For this review, use the dimensioned drawing (mm, ordinates from the lowest corner) and the shaded views. A direction names the side the tool comes from. Coordinates: 2 decimals unless noted, no trailing zeros. Loops run counter-clockwise (first coordinate to the right, second up) from the corner with the lowest first, then second, coordinate; pieces in that order, holes last. Notation, with made-up numbers: M -10.75,12.25 L 14.25,12.25 A28 cw 14.25,39.25 Z; hole C 88.25,72 d3. An arc over 180 degrees is marked long. One line per item, written item: value.
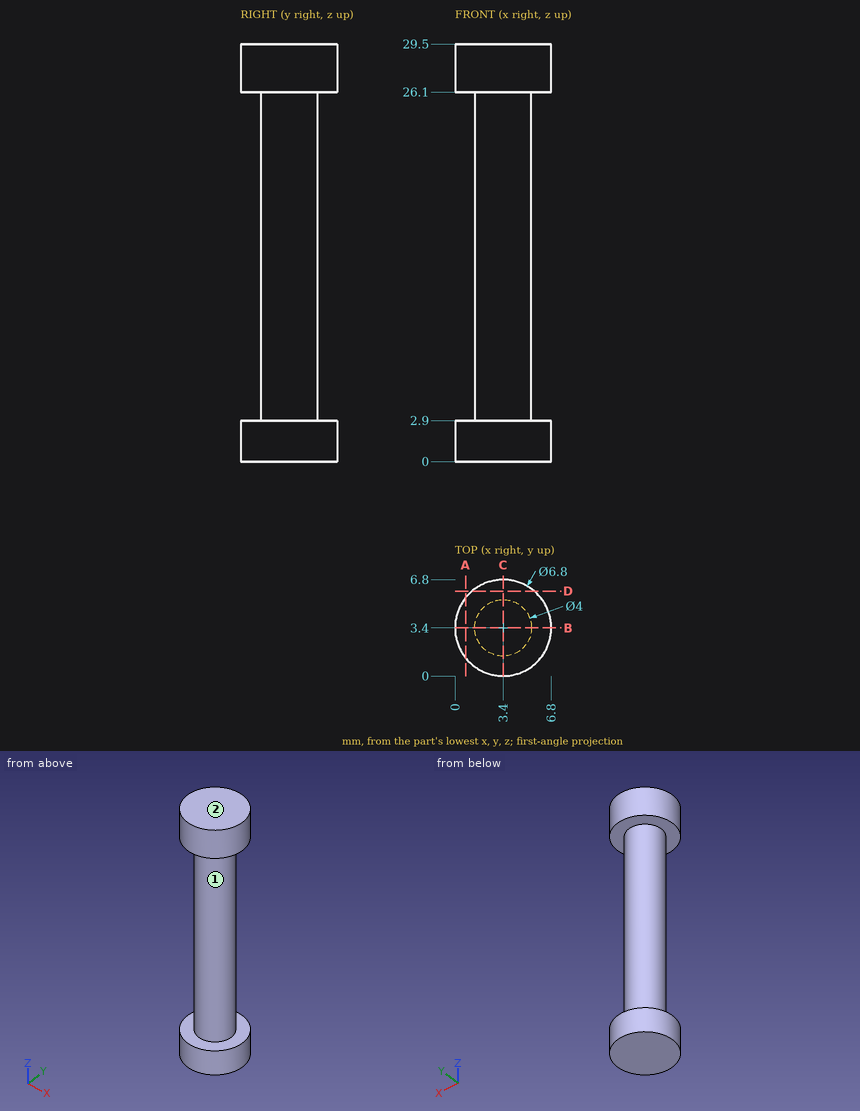
(1) Tool access review of the marked faces 1 and 2: name each direction out of +Z, -Z, +X, -X, +Y, -Y from which nothing blocks a thin tool from reaching the whole face with its end or side.
Reply:
face 1: none
face 2: +Z, +X, -X, +Y, -Y
(2) We need section D-D on y = 6. State the section outline as (x, z) points.
Reply:
outline: M 1.21,0 L 5.59,0 L 5.59,2.9 L 1.21,2.9 Z; M 1.21,26.1 L 5.59,26.1 L 5.59,29.5 L 1.21,29.5 Z
(3) We need section B-B on y = 3.4. State the section outline as (x, z) points.
Reply:
outline: M 0,0 L 6.8,0 L 6.8,2.9 L 5.4,2.9 L 5.4,26.1 L 6.8,26.1 L 6.8,29.5 L 0,29.5 L 0,26.1 L 1.4,26.1 L 1.4,2.9 L 0,2.9 Z
(4) Insertion check: pin 1 (2 mm diameter, centred on y = 5, z = 25.5, fed in from +X); pin 2 (4 mm diameter, centred on y = 5, z = 8.5, fed in from +X). Each pin has a flat end and moves straight along its axis. Give the tip position at first contact, or say it passes through.
Reply:
pin 1: stops at x = 6.7
pin 2: stops at x = 5.4
(5) To check wall thickness, follow line 1 along Z through (x, y) = (6, 2.5); line 2 along Y through (x, z) = (3.25, 11.25); line 3 along X through (y, z) = (6, 2.25). State the ranges of each line that lie inside material, in increasing order. Write a range as [from, to].
Reply:
line 1: z = [0, 2.9], [26.1, 29.5]
line 2: y = [1.41, 5.39]
line 3: x = [1.21, 5.59]
(6) We need section A-A on x = 0.75. State the section outline as (y, z) points, then the cut area to 3 significant figures.
Reply:
outline: M 1.27,0 L 5.53,0 L 5.53,2.9 L 1.27,2.9 Z; M 1.27,26.1 L 5.53,26.1 L 5.53,29.5 L 1.27,29.5 Z
area: 26.8 mm2
